Autodesk Fusion 360 part; units mm, degrees
sketch "Sketch1" plane through (0, 0, 0) normal (1, 0, 0) x (0, 0, -1)
sketch "Sketch2" plane through (0, 0, 0) normal (0, 1, 0) x (1, 0, 0)
  line L0 (10, 0) -> (32, 0)
  line L1 (42, -10) -> (42, -90)
  line L2 (32, -100) -> (10, -100)
  line L3 (0, -25) -> (-15, -25)
  line L4 (-15, -25) -> (-15, -75)
  line L5 (-15, -75) -> (0, -75)
  arc A0 (10, 0) -> (0, -10) centre (10, -10) ccw
  arc A1 (42, -10) -> (32, 0) centre (32, -10) ccw
  arc A2 (32, -100) -> (42, -90) centre (32, -90) ccw
  arc A3 (0, -90) -> (10, -100) centre (10, -90) ccw
  arc A4 (10, -7.5) -> (7.5, -10) centre (10, -10) ccw
  line L6 (7.5, -90) -> (7.5, -10)
  arc A5 (7.5, -90) -> (10, -92.5) centre (10, -90) ccw
  line L7 (32, -92.5) -> (10, -92.5)
  arc A6 (32, -92.5) -> (34.5, -90) centre (32, -90) ccw
  line L8 (34.5, -10) -> (34.5, -90)
  arc A7 (34.5, -10) -> (32, -7.5) centre (32, -10) ccw
  line L9 (10, -7.5) -> (32, -7.5)
  line L10 (0, -90) -> (0, -75)
  line L11 (0, -25) -> (0, -10)
  point P0 (42, 0)
  point P1 (0, -100)
  dimension "d11" = 42
extrude "Extrude1" add sketch "Sketch2" along normal blind 50
sketch "Sketch3" plane through (-15, 0, 0) normal (-1, 0, 0) x (0, 0, 1)
  line L0 (25, 0) -> (75, 0)
  line L1 (75, 0) -> (75, 50)
  line L2 (75, 50) -> (25, 50)
  line L3 (25, 50) -> (25, 0)
  circle A0 centre (40, 25) radius 2
  circle A1 centre (60, 25) radius 2
  dimension "d7" = 4
  dimension "d8" = 4
extrude "Extrude2" cut sketch "Sketch3" against normal blind 45 contours A0 | A1
Read the model definition and answer for the solid it produces. Units are mm, in the model's axes. A direction names the side the tool comes from. Round coordinates to 2 decimals unless told otherwise and drop trailing zeros. Write each loop counter-clockwise with the first axis right and the second up, starting at its lowest first coordinate (ties: lowest second). Pieces come first, ordered by that corner, then holes. Notation, with made-up numbers: (80, 75.5) - (139, 75.5) arc R6 ccw to (139, 80.5) - close; hole circle Ø11 at (61.25, -15). An arc over 180 degrees is marked (long way). Use a Markdown table: item, result.
(1) Straight lines are drawn through the part: line 1 along Y through (x, z) = (-8.75, 60); line 2 along X through (y, z) = (15.5, 68.5); line 3 along X through (y, z) = (3, 23.5). For each, find the intervals that lie inside material, in ascending order. Write a range as [from, to].
Reported:
| item | result |
|---|---|
| line 1 | [0, 23], [27, 50] |
| line 2 | [-15, 7.5], [34.5, 42] |
| line 3 | [0, 7.5], [34.5, 42] |
(2) The part is cut by section C-C (y = 25). Write down the section's boundary in (x, z), then the cut area to 3 significant figures.
Reported:
| item | result |
|---|---|
| outline | (-15, 25) - (0, 25) - (0, 10) arc R10 ccw to (10, 0) - (32, 0) arc R10 ccw to (42, 10) - (42, 90) arc R10 ccw to (32, 100) - (10, 100) arc R10 ccw to (0, 90) - (0, 75) - (-15, 75) - (-15, 62) - (7.5, 62) - (7.5, 90) arc R2.5 cw to (10, 92.5) - (32, 92.5) arc R2.5 cw to (34.5, 90) - (34.5, 10) arc R2.5 cw to (32, 7.5) - (10, 7.5) arc R2.5 cw to (7.5, 10) - (7.5, 38) - (-15, 38) - close; (-15, 42) - (7.5, 42) - (7.5, 58) - (-15, 58) - close |
| area | 2,390 mm2 |
(3) Each of these flat-tipped pins is pushed along its axis until it touches: pin 1 Ø4.5 at (y, z) = (16.5, 19.5) entering from -X; pin 2 Ø4.5 at (x, y) = (-11, 34) entering from -Z; pin 3 Ø12 at (x, y) = (-10, 22) entering from +Z. Where does it stop, or does it pass through?
Reported:
| item | result |
|---|---|
| pin 1 | x = 0 |
| pin 2 | z = 25 |
| pin 3 | z = 75 |
(4) The mould has two halves that part along X. Classify faces 1 (the cylindrical face through (33.748, 24.65, 8.213)), 2 (the cylindrical face through (39.15, 24.65, 96.99)), 3 (the cylindrical face through (8.252, 24.65, 91.787)), 4 (the cylindrical face through (2.85, 24.65, 3.01)): released by +X, released by -X, zero draft, split by the parting line, or undercut.
Reported:
| item | result |
|---|---|
| face 1 | undercut |
| face 2 | released by +X |
| face 3 | undercut |
| face 4 | released by -X |
(5) The part is cut by section A-A (x = 30). Write down the section's boundary in (y, z).
Reported:
| item | result |
|---|---|
| outline | (0, 0) - (50, 0) - (50, 7.5) - (0, 7.5) - close; (0, 92.5) - (50, 92.5) - (50, 100) - (0, 100) - close |
(6) Which of the six approach directions +Z, -Z, +X, -X, +Y, -Y give full straight-line access (tool end or side, diameter ignored) to faces 5 (the flat face through (0, 25, 18)), 6 (the flat face through (-8, 25, 75)), 7 (the cylindrical face through (-4, 23, 60))?
Reported:
| item | result |
|---|---|
| face 5 | -Z, -X, +Y, -Y |
| face 6 | +Z, -X, +Y, -Y |
| face 7 | -X |
(7) The part is cut by section D-D (x = -3.5). Write down the section's boundary in (y, z), then the cut area to 3 significant figures.
Reported:
| item | result |
|---|---|
| outline | (0, 25) - (50, 25) - (50, 75) - (0, 75) - close; hole circle Ø4 at (25, 40); hole circle Ø4 at (25, 60) |
| area | 2,470 mm2 |
(8) The part is cut by section B-B (z = 60). Write down the section's boundary in (x, y), then the cut area to 3 significant figures.
Reported:
| item | result |
|---|---|
| outline | (-15, 0) - (7.5, 0) - (7.5, 23) - (-15, 23) - close; (-15, 27) - (7.5, 27) - (7.5, 50) - (-15, 50) - close; (34.5, 0) - (42, 0) - (42, 50) - (34.5, 50) - close |
| area | 1,410 mm2 |
